The listing builds one solid part. Answer for the finished solid, in the listing's coordinates (mm). Face numbers are marked on the shaded views. A direction names the side the tool comes from. Give positions to 0.01 mm unless a question says otherwise; leave off trailing zeros. Loops run counter-clockwise (first coordinate to the right, second up) from the corner with the lowest first, then second, coordinate; pieces in that order, holes last. Notation, with made-up numbers: M 69.5,15.25 L 96.5,15.25 A25 ccw 96.5,52.25 Z; hole C -5,-7.75 d4. An arc over 180 degrees is marked long. Return JSON: item names as keys, results as strings.
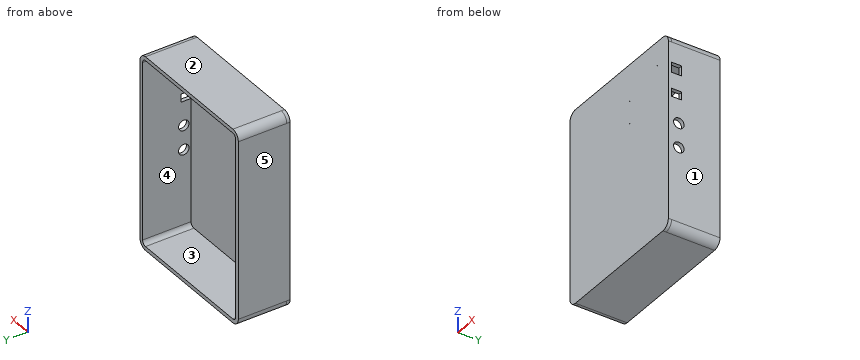
from build123d import *

# Parameters (mm, degrees)
SKETCH1_W               = 180
SKETCH1_H               = 240
BOSS_EXTRUDE1_DEPTH     = 4
FILLET1_R               = 10
BOSS_EXTRUDE2_DEPTH     = 60
SKETCH3_R               = 0.5
CUT_EXTRUDE1_DEPTH      = 61
CUT_EXTRUDE1_DEPTH_BACK = 5
SKETCH4_W               = 15
SKETCH4_H               = 12.5
SKETCH4_W_2             = 20
SKETCH4_H_2             = 10
CUT_EXTRUDE2_DEPTH      = 12.6
SKETCH5_R               = 6.5
CUT_EXTRUDE3_DEPTH      = 12.6


with BuildPart() as part:
    # Sketch1 → Boss-Extrude1 (new body)
    with BuildSketch(Plane(origin=(0, 0, 0), x_dir=(1, 0, 0), z_dir=(0, 1, 0))):
        with Locations((90, 120)):
            Rectangle(SKETCH1_W, SKETCH1_H)
    extrude(amount=BOSS_EXTRUDE1_DEPTH)

    # Fillet1
    fillet1_edges = [part.edges().sort_by_distance(p)[0] for p in [
        (0, 2, -240),
        (180, 2, -240),
        (180, 2, 0),
        (0, 2, 0),
    ]]
    fillet(fillet1_edges, radius=FILLET1_R)

    # Sketch2 → Boss-Extrude2 (add)
    with BuildSketch(Plane(origin=(0, 4, 0), x_dir=(1, 0, 0), z_dir=(0, 1, 0))):
        with BuildLine():
            Line((170, 240), (10, 240))
            ThreePointArc((10, 240), (2.928932188, 237.071067812), (0, 230))
            Line((0, 230), (0, 10))
            ThreePointArc((0, 10), (2.928932188, 2.928932188), (10, 0))
            Line((10, 0), (170, 0))
            ThreePointArc((170, 0), (177.071067812, 2.928932188), (180, 10))
            Line((180, 10), (180, 230))
            ThreePointArc((180, 230), (177.071067812, 237.071067812), (170, 240))
        make_face()
        with BuildLine():
            Line((170, 235.2), (10, 235.2))
            ThreePointArc((10, 235.2), (6.323044738, 233.676955262), (4.8, 230))
            Line((4.8, 230), (4.8, 10))
            ThreePointArc((4.8, 10), (6.323044738, 6.323044738), (10, 4.8))
            Line((10, 4.8), (170, 4.8))
            ThreePointArc((170, 4.8), (173.676955262, 6.323044738), (175.2, 10))
            Line((175.2, 10), (175.2, 230))
            ThreePointArc((175.2, 230), (173.676955262, 233.676955262), (170, 235.2))
        make_face(mode=Mode.SUBTRACT)
    extrude(amount=BOSS_EXTRUDE2_DEPTH)

    # Sketch3 → Cut-Extrude1 (cut, two sides)
    with BuildSketch(Plane(origin=(0, 4, 0), x_dir=(1, 0, 0), z_dir=(0, 1, 0))) as cut_extrude1_sk:
        with Locations((159.96, 29.8)):
            Circle(SKETCH3_R)
        with Locations((109.7, 45.3)):
            Circle(SKETCH3_R)
        with Locations((109.7, 73.3)):
            Circle(SKETCH3_R)
    extrude(amount=CUT_EXTRUDE1_DEPTH, mode=Mode.SUBTRACT)
    extrude(cut_extrude1_sk.sketch, amount=-CUT_EXTRUDE1_DEPTH_BACK, mode=Mode.SUBTRACT)

    # Sketch4 → Cut-Extrude2 (cut)
    with BuildSketch(Plane(origin=(0, 4, 0), x_dir=(1, 0, 0), z_dir=(0, 1, 0))):
        with Locations((175.2, 41.25)):
            Rectangle(SKETCH4_W, SKETCH4_H)
        with Locations((175.2, 72.29)):
            Rectangle(SKETCH4_W_2, SKETCH4_H_2)
    extrude(amount=CUT_EXTRUDE2_DEPTH, mode=Mode.SUBTRACT)

    # Sketch5 → Cut-Extrude3 (cut)
    with BuildSketch(Plane(origin=(180, 0, 0), x_dir=(0, 0, -1), z_dir=(1, 0, 0))):
        with Locations((107.29, 13)):
            Circle(SKETCH5_R)
        with Locations((137.29, 13)):
            Circle(SKETCH5_R)
    extrude(amount=-CUT_EXTRUDE3_DEPTH, mode=Mode.SUBTRACT)


solid = part.part
(1) The part is cut by section C-C (z = -80). Determine the outline of the cut face in (x, y).
Values follow:
{"outline": "M 0,0 L 180,0 L 180,64 L 175.2,64 L 175.2,4 L 4.8,4 L 4.8,64 L 0,64 Z"}
(2) Given pin 1 (1.4 mm diameter, centred on x = 178.5, y = 12.5, fed in from +Z); pin 2 (4 mm diameter, centred on x = 178.5, y = 9.5, fed in from -Z); pin 3 (4 mm diameter, centred on x = 177, y = 9, fed in from -Z), each flat-ended and moving along its own axis, determine where each tip first touches the part or whether it passes through.
Values follow:
{"pin 1": "z = -3.74", "pin 2": "z = -237.6", "pin 3": "z = -238.66"}
(3) The part is cut by section D-D (y = 58.5). Determine the outline of the cut face in (x, z).
Values follow:
{"outline": "M 0,-230 A10 ccw 10,-240 L 170,-240 A10 ccw 180,-230 L 180,-10 A10 ccw 170,0 L 10,0 A10 ccw 0,-10 Z; hole M 4.8,-230 A5.2 ccw 10,-235.2 L 170,-235.2 A5.2 ccw 175.2,-230 L 175.2,-10 A5.2 ccw 170,-4.8 L 10,-4.8 A5.2 ccw 4.8,-10 Z"}
(4) Straight lines are drawn through the part: line 1 along X through (y, z) = (2.7, -73.3); line 2 along X through (y, z) = (40, -22.5); line 3 along Z through (x, y) = (87.5, 42.5). For each, find the intervals that lie inside material, in ascending order.
Values follow:
{"line 1": "0 to 109.2, 110.2 to 180", "line 2": "0 to 4.8, 175.2 to 180", "line 3": "-240 to -235.2, -4.8 to 0"}
(5) The part is cut by section B-B (y = 9). Give the number of separate pieces and of enclosed holes in the cut face, and give its area (3 significant figures).
Values follow:
{"separate pieces": "4", "enclosed holes": "0", "area": "3,670 mm²"}
(6) Determine the mould class of the marked faces 1, 2 and 3 for opening direction X: released by +X, released by -X, zero draft, split by the parting line, or undercut.
Values follow:
{"face 1": "released by +X", "face 2": "zero draft", "face 3": "undercut"}
(7) A tool of negligible diameter and unlimited length cuts with its end or side. For the marked faces 4 and 5, from which of +Z, -Z, +X, -X, +Y, -Y can it reach the whole face along a straight path? Write none if from no direction.
Values follow:
{"face 4": "+Y", "face 5": "+Z, -Z, -X, +Y, -Y"}
(8) The part is cut by section A-A (z = -137.29). Determine the outline of the cut face in (x, y), and give its area (3 significant figures).
Values follow:
{"outline": "M 0,0 L 180,0 L 180,6.5 L 175.2,6.5 L 175.2,4 L 4.8,4 L 4.8,64 L 0,64 Z; M 175.2,19.5 L 180,19.5 L 180,64 L 175.2,64 Z", "area": "1,230 mm²"}
